from build123d import *

# Parameters (mm, degrees)
SKETCH1_W           = 30
SKETCH1_H           = 64
BOSS_EXTRUDE1_DEPTH = 3
SKETCH2_R           = 4.5
SKETCH2_R_2         = 6
CUT_EXTRUDE1_DEPTH  = 3
SKETCH4_W           = 30
SKETCH4_H           = 3
BOSS_EXTRUDE3_DEPTH = 15
SKETCH5_R           = 1.25
CUT_EXTRUDE2_DEPTH  = 15


with BuildPart() as part:
    # Sketch1 → Boss-Extrude1 (new body)
    with BuildSketch(Plane.XY):
        with Locations((-16.801372712, 6.218640229)):
            Rectangle(SKETCH1_W, SKETCH1_H)
    extrude(amount=BOSS_EXTRUDE1_DEPTH)

    # Sketch2 → Cut-Extrude1 (cut)
    with BuildSketch(Plane.XY.offset(3)):
        with Locations((-16.801372712, 22.218640229)):
            Circle(SKETCH2_R)
        with Locations((-16.801372712, -9.781359771)):
            Circle(SKETCH2_R_2)
    extrude(amount=-CUT_EXTRUDE1_DEPTH, mode=Mode.SUBTRACT)

    # Sketch4 → Boss-Extrude3 (add)
    with BuildSketch(Plane(origin=(0, 0, 0), x_dir=(-1, 0, 0), z_dir=(0, 0, -1))):
        with Locations((16.801372712, -24.281359771)):
            Rectangle(SKETCH4_W, SKETCH4_H)
    extrude(amount=BOSS_EXTRUDE3_DEPTH)

    # Sketch5 → Cut-Extrude2 (cut)
    with BuildSketch(Plane(origin=(0, -22.781359771, 0), x_dir=(1, 0, 0), z_dir=(0, 1, 0))):
        with Locations((-9.801372712, 7.5)):
            Circle(SKETCH5_R)
        with Locations((-23.801372712, 7.5)):
            Circle(SKETCH5_R)
    extrude(amount=-CUT_EXTRUDE2_DEPTH, mode=Mode.SUBTRACT)


solid = part.part
Geometry check sheet. Reference: the model listing, model coordinates, mm. A direction names the side the tool comes from. Round coordinates to 2 decimals unless told otherwise and drop trailing zeros. Write each loop counter-clockwise with the first axis right and the second up, starting at its lowest first coordinate (ties: lowest second). Pieces come first, ordered by that corner, then holes. Notation, with made-up numbers: (52.25, -19) - (58.25, -19) arc R16 cw to (58.25, 9) - close; hole circle Ø6 at (10.5, 69.5). An arc over 180 degrees is marked (long way). One line per item, written item: value.
1. Depth check by flat-ended pin: pin 1 Ø3 at (x, y) = (-15, -16.5) entering from -Z; pin 2 Ø2 at (x, z) = (-23.8, -7.5) entering from +Y; pin 3 Ø1 at (x, z) = (-12.5, -3.5) entering from +Y. Enter the tip coordinate at first touch or a pass-through.
The answers:
pin 1: stops at z = 0
pin 2: passes through
pin 3: stops at y = -22.78
2. Cross-section at A-A on z = -7.5. Record the boundary of the cut face in (x, y).
The answers:
outline: (-31.8, -25.78) - (-25.05, -25.78) - (-25.05, -22.78) - (-31.8, -22.78) - close; (-22.55, -25.78) - (-11.05, -25.78) - (-11.05, -22.78) - (-22.55, -22.78) - close; (-8.55, -25.78) - (-1.8, -25.78) - (-1.8, -22.78) - (-8.55, -22.78) - close
3. Scan lines: L1, parallel to X at y = -25.05, z = -7.5; L2, parallel to Y at x = -17, z = 1.5; L3, parallel to Y at x = -25, z = -9.75. Record each from-to range of solid material in increasing order.
The answers:
L1: x = -31.8 to -25.05, -22.55 to -11.05, -8.55 to -1.8
L2: y = -25.78 to -15.78, -3.78 to 17.72, 26.71 to 38.22
L3: y = -25.78 to -22.78
4. Set-up check for faces 5 (the face through (-10.793, -24.26, -6.739)), 6 (the face through (-17, 8, 0)): record each of +Z, -Z, +X, -X, +Y, -Y from which the full face is reachable in a straight line by a thin tool's end or side.
The answers:
face 5: +Y, -Y
face 6: -Z, +X, -X, +Y
5. Cross-section at C-C on x = -20.25. Record the boundary of the cut face in (y, z).
The answers:
outline: (-25.78, -15) - (-22.78, -15) - (-22.78, 0) - (-14.69, 0) - (-14.69, 3) - (-25.78, 3) - close; (-4.87, 0) - (19.33, 0) - (19.33, 3) - (-4.87, 3) - close; (25.11, 0) - (38.22, 0) - (38.22, 3) - (25.11, 3) - close
6. Cross-section at D-D on y = 13. Record the boundary of the cut face in (x, z), and give its area (3 significant figures).
The answers:
outline: (-31.8, 0) - (-1.8, 0) - (-1.8, 3) - (-31.8, 3) - close
area: 90.0 mm^2
7. Mould release check, pull along Z, two halves, no side actions. Record for faces 1 (the face through (-25.05, -24.26, -7.55)), 2 (the face through (-17, 38.219, 1)), 3 (the face through (-17, 7, 3)), 4 (the face through (-17, -24, -15)): released by +Z, released by -Z, zero draft, split by the parting line, or undercut.
The answers:
face 1: undercut
face 2: zero draft
face 3: released by +Z
face 4: released by -Z
8. Cross-section at B-B on x = -4.25. Record the boundary of the cut face in (y, z), and give its area (3 significant figures).
The answers:
outline: (-25.78, -15) - (-22.78, -15) - (-22.78, 0) - (38.22, 0) - (38.22, 3) - (-25.78, 3) - close
area: 237 mm^2
